Autodesk Inventor part; units mm, degrees
ref_plane "YZ Plane" through (0, 0, 0) normal (1, 0, 0) x (0, 1, 0)
ref_plane "XZ Plane" through (0, 0, 0) normal (0, 1, 0) x (-1, 0, 0)
ref_plane "XY Plane" through (0, 0, 0) normal (0, 0, 1) x (1, 0, 0)
sketch "Sketch1" plane through (0, 0, 0) normal (0, 0, 1) x (1, 0, 0)
  circle A0 centre (0, 0) radius 3.5
  circle A1 centre (8.25, 0) radius 1.55
  circle A2 centre (-8.25, 0) radius 1.55
  line L0 (0, 0) -> (0, 12.5)
  line L1 (0, 12.5) -> (12.5, 12.5)
  line L2 (12.5, 0) -> (12.5, 12.5)
  line L3 (0, 12.5) -> (-12.5, 12.5)
  line L4 (-12.5, 12.5) -> (-12.5, 0)
  arc A3 (-12.5, 0) -> (12.5, 0) centre (0, 0) ccw
  dimension "d0" = 7
  dimension "d4" = 3.1
  dimension "d5" = 3.1
  dimension "d9" = 12.5
  dimension "d10" = 12.5
extrude "Extrusion1" add sketch "Sketch1" along normal blind 2.5
sketch "Sketch2" plane through (0, 0, 2.5) normal (0, 0, 1) x (1, 0, 0)
  line L0 (-12.5, 12.5) -> (-12.5, 0)
  line L1 (12.5, 0) -> (12.5, 12.5)
  line L2 (-12.5, 12.5) -> (12.5, 12.5)
  line L3 (12.5, 14.9) -> (-12.5, 14.9)
  line L4 (-12.5, 12.5) -> (-20.5, 12.5)
  line L5 (-20.5, 12.5) -> (-20.5, 14.9)
  line L6 (-20.5, 14.9) -> (-12.5, 14.9)
  line L7 (12.5, 12.5) -> (20.5, 12.5)
  line L8 (20.5, 12.5) -> (20.5, 14.9)
  line L9 (20.5, 14.9) -> (12.5, 14.9)
  point P0 (0, 0)
  dimension "d14" = 8
  dimension "d15" = 2.4
  dimension "d17" = 2.4
extrude "Extrusion2" add sketch "Sketch2" against normal blind 15
sketch "Sketch3" plane through (0, 0, 2.5) normal (0, 0, 1) x (1, 0, 0)
  arc A0 (-12.5, 0) -> (12.5, 0) centre (0, 0) ccw
  line L0 (20.5, 12.5) -> (-20.5, 12.5)
  line L1 (12.5, 12.5) -> (-12.5, 12.5)
  arc A1 (-12.5, 0) -> (-20.5, 12.5) centre (-27.4799, -0.7771) ccw
  arc A2 (20.5, 12.5) -> (12.5, 0) centre (27.4799, -0.7771) ccw
  line L2 (-20.5, 12.5) -> (-12.5, 12.5)
  line L3 (-12.5, 12.5) -> (-12.5, 0)
  line L4 (-12.5, 0) -> (-12.5, 12.5)
  line L5 (12.5, 0) -> (12.5, 12.5)
  line L6 (12.5, 0) -> (12.5, 12.5)
  line L7 (12.5, 12.5) -> (20.5, 12.5)
  dimension "d20" = 15
  dimension "d21" = 15
extrude "Extrusion3" add sketch "Sketch3" against normal up to surface (2.5 mm away) contours A1 L0 L3 | L5 L0 A2
sketch "Sketch4" plane through (-20.5, 14.9, 2.5) normal (0, 1, 0) x (1, 0, 0)
  line L0 (41, 15) -> (0, 15)
  line L1 (0, 0) -> (0, 15)
  line L2 (41, 0) -> (41, 15)
  line L3 (41, 7.5) -> (36, 7.5)
  circle A0 centre (5, 7.5) radius 1.55
  circle A1 centre (36, 7.5) radius 1.55
  point P0 (20.5, 2.5)
  dimension "d27" = 3.1
  dimension "d28" = 3.1
extrude "Extrusion4" cut sketch "Sketch4" against normal blind 10
properties part number "main_motor_mount" material "Prusament PETG"
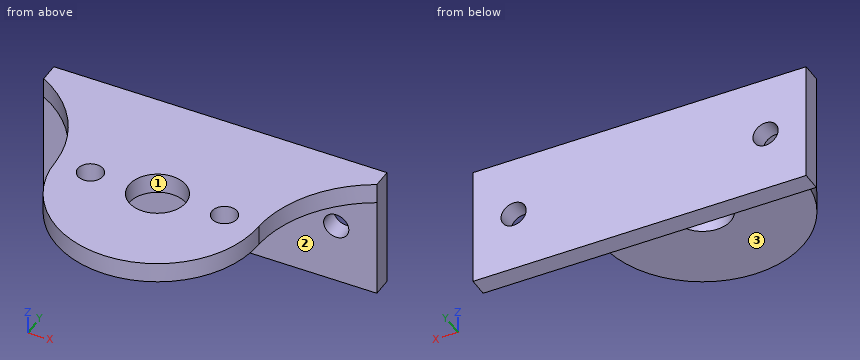
For this review, take the finished solid that the model builds, in its own axes (mm). Face numbers are marked on the shaded views. Give positions to 0.01 mm unless a question says otherwise; leave off trailing zeros. Write each loop counter-clockwise with the first axis right and the second up, starting at its lowest first coordinate (ties: lowest second). Pieces come first, ordered by that corner, then holes.
Item 1: Take a section at B-B (x = 0). Give the boundary of the cut face in (y, z), and give its area (3 significant figures).
Item 2: Take a section at C-C (z = 0.75). Give the boundary of the cut face in (x, y).
Item 3: Take a section at A-A (z = -5). Give the boundary of the cut face in (x, y).
Item 4: Take a section at D-D (x = -9). Give the boundary of the cut face in (y, z), and give its area (3 significant figures).
Item 5: The part is to be moulded in two halves that separate along Y. For the marked faces 1, 2 and 3, say which applies: +Y half, -Y half, draft (parallel to the pull), parting line (faces both ways), or undercut.
Item 6: Wall thickness on probe 1 along X at (y, z) = (13, -5); probe 2 along Y at (x, z) = (0, 1.85); probe 3 along Z at (x, y) = (14.5, 7.25): over which ranges is each line inside the solid? List them lowest first.
Item 7: Insertion check: P1, Ø4, axis at x = -7.5, z = -7, coming from the -Y side; P2, Ø3, axis at x = -6, y = 5, coming from the -Z side. Each pin has a flat end and moves straight along its axis. Give the tip position at first contact, or say it passes through.
Established:
1. outline: (-12.5, 0) - (-3.5, 0) - (-3.5, 2.5) - (-12.5, 2.5) - close; (3.5, 0) - (12.5, 0) - (12.5, -12.5) - (14.9, -12.5) - (14.9, 2.5) - (3.5, 2.5) - close
1. area: 81.0 mm2
2. outline: (-20.5, 12.5) arc R15 cw to (-12.5, 0) arc R12.5 ccw to (12.5, 0) arc R15 cw to (20.5, 12.5) - (20.5, 14.9) - (-20.5, 14.9) - close; hole circle Ø3.1 at (-8.25, 0); hole circle Ø7 at (0, 0); hole circle Ø3.1 at (8.25, 0)
3. outline: (-20.5, 12.5) - (-17.05, 12.5) - (-17.05, 14.9) - (-20.5, 14.9) - close; (-13.95, 12.5) - (13.95, 12.5) - (13.95, 14.9) - (-13.95, 14.9) - close; (17.05, 12.5) - (20.5, 12.5) - (20.5, 14.9) - (17.05, 14.9) - close
4. outline: (-8.67, 0) - (-1.36, 0) - (-1.36, 2.5) - (-8.67, 2.5) - close; (1.36, 0) - (12.5, 0) - (12.5, -12.5) - (14.9, -12.5) - (14.9, 2.5) - (1.36, 2.5) - close
4. area: 82.2 mm2
5. face 1: undercut
5. face 2: -Y half
5. face 3: draft
6. probe 1: x = -20.5 to -17.05, -13.95 to 13.95, 17.05 to 20.5
6. probe 2: y = -12.5 to -3.5, 3.5 to 14.9
6. probe 3: z = 0 to 2.5
7. P1: stops at y = 12.5
7. P2: stops at z = 0
